from build123d import *

# Parameters (mm, degrees)
SKETCH_1_R                             = 1.1
PCB20X20_T1P6_2NPTH_D2P2_PITCH15_DEPTH = 1.6


with BuildPart() as part:
    # 草图1 → PCB20x20_T1p6_2NPTH_D2p2_pitch15 (new body)
    with BuildSketch(Plane.XY):
        with BuildLine():
            Line((-9, -10), (9, -10))
            ThreePointArc((9, -10), (9.707106781, -9.707106781), (10, -9))
            Line((10, -9), (10, 9))
            ThreePointArc((10, 9), (9.707106781, 9.707106781), (9, 10))
            Line((9, 10), (-9, 10))
            ThreePointArc((-9, 10), (-9.707106781, 9.707106781), (-10, 9))
            Line((-10, 9), (-10, -9))
            ThreePointArc((-10, -9), (-9.707106781, -9.707106781), (-9, -10))
        make_face()
        with Locations((0, -7.5)):
            Circle(SKETCH_1_R, mode=Mode.SUBTRACT)
        with Locations((0, 7.5)):
            Circle(SKETCH_1_R, mode=Mode.SUBTRACT)
    extrude(amount=PCB20X20_T1P6_2NPTH_D2P2_PITCH15_DEPTH)


solid = part.part
Input: part model. Units: mm. Frame: model coordinates. Give positions to 0.01 mm unless a question says otherwise; leave off trailing zeros. Write each loop counter-clockwise with the first axis right and the second up, starting at its lowest first coordinate (ties: lowest second). Pieces come first, ordered by that corner, then holes. Notation, with made-up numbers: M 58,56 L 108,56 A20 cw 108,62 Z; hole C 16.25,56 d6. An arc over 180 degrees is marked long. Write item = value, one per line. Start each with the question number.
1) Draft query along X for faces 1 (the cylindrical face through (-9.715, -9.699, 0.789)), 2 (the cylindrical face through (-0.238, -8.574, 0.789)), 3 (the cylindrical face through (9.715, 9.699, 0.789)). Return one class per face: +X half, -X half, draft (parallel to the pull), parting line (faces both ways), or undercut.
2) Cut plane B-B on z = 0.3. Return the cut outline in (x, y), then the cut area to 3 significant figures.
3) Cut plane A-A on x = 0. Return the cut outline in (y, z), then the cut area to 3 significant figures.
4) Material intervals for line 1 along Y through (x, z) = (0, 0.55); line 2 along Y through (x, z) = (1, 1.35); line 3 along X through (y, z) = (-8.25, 0.2), sorted ascending. Write a range as [from, to].
5) Cut plane C-C on y = -7.5. Return the cut outline in (x, z).
6) First-contact query: pin 1 Ø12 at (x, y) = (-2, -4.5) entering from -Z. Flat tip, straight axial feed; report the tip coordinate or a pass-through.
Solved:
q1.face_1 = -X half
q1.face_2 = undercut
q1.face_3 = +X half
q2.outline = M -10,-9 A1 ccw -9,-10 L 9,-10 A1 ccw 10,-9 L 10,9 A1 ccw 9,10 L -9,10 A1 ccw -10,9 Z; hole C 0,-7.5 d2.2; hole C 0,7.5 d2.2
q2.area = 392 mm2
q3.outline = M -10,0 L -8.6,0 L -8.6,1.6 L -10,1.6 Z; M -6.4,0 L 6.4,0 L 6.4,1.6 L -6.4,1.6 Z; M 8.6,0 L 10,0 L 10,1.6 L 8.6,1.6 Z
q3.area = 25.0 mm2
q4.line_1 = [-10, -8.6], [-6.4, 6.4], [8.6, 10]
q4.line_2 = [-10, -7.96], [-7.04, 7.04], [7.96, 10]
q4.line_3 = [-10, -0.8], [0.8, 10]
q5.outline = M -10,0 L -1.1,0 L -1.1,1.6 L -10,1.6 Z; M 1.1,0 L 10,0 L 10,1.6 L 1.1,1.6 Z
q6.pin_1 = 0
